Source: CAD feature listing. Evaluate the final solid. Frame: model axes, mm. Face numbers are marked on the shaded views. A direction names the side the tool comes from. Round coordinates to 2 decimals unless told otherwise and drop trailing zeros. Loops run counter-clockwise (first coordinate to the right, second up) from the corner with the lowest first, then second, coordinate; pieces in that order, holes last. Notation, with made-up numbers: (80.25, -24.75) - (121.25, -24.75) arc R17 ccw to (121.25, -4.75) - close; hole circle Ø11 at (47.5, 79.5). An arc over 180 degrees is marked (long way). One line per question, with ' | ' between items.
from build123d import *

# Parameters (mm, degrees)
SKETCH1_R           = 3.302
SKETCH1_R_2         = 3.175
SKETCH1_W           = 36.231873889
SKETCH1_H           = 34.54456272
BOSS_EXTRUDE1_DEPTH = 2.54
SKETCH3_W           = 9.144
SKETCH3_H           = 3.81
BOSS_EXTRUDE2_DEPTH = 8.89
FILLET1_R           = 2.54


with BuildPart() as part:
    # Sketch1 → Boss-Extrude1 (new body)
    with BuildSketch(Plane.XY):
        with BuildLine():
            Line((19.05, 113.03), (19.05, 107.95))
            ThreePointArc((19.05, 107.95), (19.793948776, 106.153948776), (21.59, 105.41))
            Line((21.59, 105.41), (69.85, 105.41))
            Line((69.85, 105.41), (69.85, -3.81))
            Line((69.85, -3.81), (21.59, -3.81))
            ThreePointArc((21.59, -3.81), (19.793948776, -4.553948776), (19.05, -6.35))
            Line((19.05, -6.35), (19.05, -11.43))
            ThreePointArc((19.05, -11.43), (18.306051224, -13.226051224), (16.51, -13.97))
            Line((16.51, -13.97), (11.43, -13.97))
            ThreePointArc((11.43, -13.97), (9.633948776, -13.226051224), (8.89, -11.43))
            Line((8.89, -11.43), (8.89, -6.35))
            ThreePointArc((8.89, -6.35), (8.146051224, -4.553948776), (6.35, -3.81))
            Line((6.35, -3.81), (-3.81, -3.81))
            Line((-3.81, -3.81), (-3.81, 105.41))
            Line((-3.81, 105.41), (6.35, 105.41))
            ThreePointArc((6.35, 105.41), (8.146051224, 106.153948776), (8.89, 107.95))
            Line((8.89, 107.95), (8.89, 113.03))
            ThreePointArc((8.89, 113.03), (9.633948776, 114.826051224), (11.43, 115.57))
            Line((11.43, 115.57), (16.51, 115.57))
            ThreePointArc((16.51, 115.57), (18.306051224, 114.826051224), (19.05, 113.03))
        make_face()
        with Locations((13.97, 110.49)):
            Circle(SKETCH1_R, mode=Mode.SUBTRACT)
        with Locations((13.97, -8.89)):
            Circle(SKETCH1_R, mode=Mode.SUBTRACT)
        with Locations((14.607116803, 73.380830868)):
            Circle(SKETCH1_R_2, mode=Mode.SUBTRACT)
        with Locations((42.844063056, 79.24771864)):
            Rectangle(SKETCH1_W, SKETCH1_H, mode=Mode.SUBTRACT)
    extrude(amount=BOSS_EXTRUDE1_DEPTH)

    # Sketch3 → Boss-Extrude2 (add)
    with BuildSketch(Plane(origin=(0, 0, 0), x_dir=(-1, 0, 0), z_dir=(0, 0, -1))):
        with Locations((-42.418, -1.905)):
            Rectangle(SKETCH3_W, SKETCH3_H)
    extrude(amount=BOSS_EXTRUDE2_DEPTH)

    # Fillet1
    fillet1_edges = [part.edges().sort_by_distance(p)[0] for p in [
        (24.728126111, 61.97543728, 1.27),
        (60.96, 61.97543728, 1.27),
        (60.96, 96.52, 1.27),
        (24.728126111, 96.52, 1.27),
    ]]
    fillet(fillet1_edges, radius=FILLET1_R)


solid = part.part
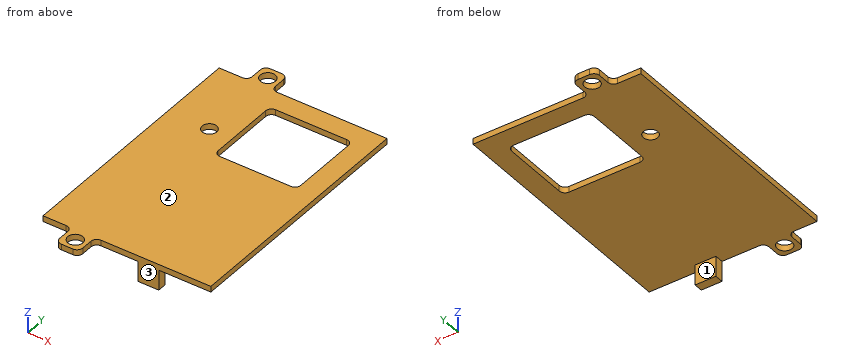
1. Section query D-D, the plane y = 88. Return loops of the section in (x, z).
Worked out:
outline: (-3.81, 0) - (24.73, 0) - (24.73, 2.54) - (-3.81, 2.54) - close; (60.96, 0) - (69.85, 0) - (69.85, 2.54) - (60.96, 2.54) - close
2. Access query for the marked faces 1, 2 and 3. Directions: +Z, -Z, +X, -X, +Y, -Y. A direction counts if a zero-diameter tool reaches every point of the face in a straight line with its end or side. Return the directions, or none.
Worked out:
face 1: -Z, +X, -X, +Y | face 2: +Z, +X, -X, +Y, -Y | face 3: +Z, -Z, +X, -Y
3. Contact query for flat-ended pins moving along their axis: P1, Ø2, axis at x = 3.5, z = 1, coming from the -Y side; P2, Ø7.5, axis at x = 13.97, y = 110.49, coming from the -Z side; P3, Ø0.8, axis at y = -7.5, z = 1, coming from the +X side; P4, Ø12, axis at x = 54.5, y = 80.5, coming from the -Z side. Output: stop coordinate, or through.
Worked out:
P1: stops at y = -3.81 | P2: stops at z = 0 | P3: stops at x = 19.05 | P4: passes through
4. Section query B-B, the plane y = 110.49. Return loops of the section in (x, z).
Worked out:
outline: (8.89, 0) - (10.67, 0) - (10.67, 2.54) - (8.89, 2.54) - close; (17.27, 0) - (19.05, 0) - (19.05, 2.54) - (17.27, 2.54) - close
5. Material intervals for probe 1 along Y at (x, z) = (13.97, 0.85); probe 2 along Y at (x, z) = (47, 1.75); probe 3 along Z at (x, y) = (22, 80.5), sorted ascending.
Worked out:
probe 1: y = -13.97 to -12.19, -5.59 to 70.27, 76.49 to 107.19, 113.79 to 115.57 | probe 2: y = -3.81 to 61.98, 96.52 to 105.41 | probe 3: z = 0 to 2.54
6. Section query C-C, the plane x = 15. Return loops of the section in (y, z).
Worked out:
outline: (-13.97, 0) - (-12.03, 0) - (-12.03, 2.54) - (-13.97, 2.54) - close; (-5.75, 0) - (70.23, 0) - (70.23, 2.54) - (-5.75, 2.54) - close; (76.53, 0) - (107.35, 0) - (107.35, 2.54) - (76.53, 2.54) - close; (113.63, 0) - (115.57, 0) - (115.57, 2.54) - (113.63, 2.54) - close
7. Section query A-A, the plane x = 45. Return loops of the section in (y, z).
Worked out:
outline: (-3.81, -8.89) - (0, -8.89) - (0, 0) - (61.98, 0) - (61.98, 2.54) - (-3.81, 2.54) - close; (96.52, 0) - (105.41, 0) - (105.41, 2.54) - (96.52, 2.54) - close
